Verification items for the finished model (mm, model axes). A direction names the side the tool comes from. Coordinates: 2 decimals unless noted, no trailing zeros. Write each loop counter-clockwise with the first axis right and the second up, starting at its lowest first coordinate (ties: lowest second). Pieces come first, ordered by that corner, then holes. Notation, with made-up numbers: (-21.5, 29.5) -> (-5.5, 29.5) arc R16 ccw to (-5.5, 41.5) -> close; hole circle Ø2 at (-23.5, -5). An arc over 180 degrees is marked (long way). Answer in a Markdown table with one row per item.
```python
from build123d import *

# Parameters (mm, degrees)
F0_W     = 65
F0_H     = 61
F1_DEPTH = 17.5
F2_T     = -2
F3_R     = 1.2
F4_W     = 0.8
F4_H     = 30.2
F5_DEPTH = 5
F7_DEPTH = 2


with BuildPart() as f1:
    # F0 (on Top) → F1 (new body)
    with BuildSketch(Plane.XY):
        Rectangle(F0_W, F0_H)
    extrude(amount=F1_DEPTH)

    # F2
    f2_openings = [f1.faces().sort_by_distance(p)[0] for p in [
        (0, 0, 17.5),
    ]]
    offset(amount=F2_T, openings=f2_openings)

    # F3
    f3_edges = [f1.edges().sort_by_distance(p)[0] for p in [
        (32.5, -30.5, 8.75),
        (32.5, 30.5, 8.75),
        (-32.5, 30.5, 8.75),
        (-32.5, -30.5, 8.75),
        (0, -30.5, 0),
        (-32.5, 0, 0),
        (32.5, 0, 0),
        (0, 30.5, 0),
    ]]
    fillet(f3_edges, radius=F3_R)

    # F4 (on face) → F5 (join)
    with BuildSketch(Plane.XY.offset(2)):
        Polygon((30.5, 2.5), (-30.5, 2.5), (-30.5, 1.7), (-1.3, 1.7), (-0.5, 1.7), (30.5, 1.7), align=None)
        with Locations((-0.9, -13.4)):
            Rectangle(F4_W, F4_H)
    extrude(amount=F5_DEPTH)

    # F6 (on face) → F7 (cut, through all)
    with BuildSketch(Plane(origin=(-32.5, 0, 0), x_dir=(0, -1, 0), z_dir=(-1, 0, 0))):
        Polygon((-20.3, 4.2), (-28.3, 4.2), (-27.3, 2.2), (-21.3, 2.2), align=None)
    extrude(amount=-F7_DEPTH, mode=Mode.SUBTRACT)


solid = f1.part
```
1. Depth check by flat-ended pin: P1, Ø1, axis at x = -22.5, y = 20, coming from the +Z side; P2, Ø3, axis at x = 2, y = 2.5, coming from the +Z side. Enter the tip coordinate at first touch or a pass-through.
Geometry says:
| item | result |
|---|---|
| P1 | z = 2 |
| P2 | z = 7 |
2. Mould release check, pull along Y, two halves, no side actions. Record for faces 4 (the flat face through (0, 30.5, 9)), 5 (the flat face through (0, 0, 0)), 6 (the flat face through (-31.5, 20.8, 3.2)): released by +Y, released by -Y, zero draft, split by the parting line, or undercut.
Geometry says:
| item | result |
|---|---|
| face 4 | released by +Y |
| face 5 | zero draft |
| face 6 | undercut |
3. Tool access check on faces 1 (the flat face through (0, -28.5, 10)), 2 (the flat face through (-32, 24, 4.2)), 3 (the flat face through (-32.5, 0, 9)). Record the directions out of +Z, -Z, +X, -X, +Y, -Y that give a thin tool (end or side, any length) a straight path to the whole face; none if there is none.
Geometry says:
| item | result |
|---|---|
| face 1 | +Z |
| face 2 | -X |
| face 3 | +Z, -Z, -X, +Y, -Y |
4. Section check D-D, the plane z = 11.5. Record the boundary of the cut face in (x, y).
Geometry says:
| item | result |
|---|---|
| outline | (-32.5, -29.3) arc R1.2 ccw to (-31.3, -30.5) -> (31.3, -30.5) arc R1.2 ccw to (32.5, -29.3) -> (32.5, 29.3) arc R1.2 ccw to (31.3, 30.5) -> (-31.3, 30.5) arc R1.2 ccw to (-32.5, 29.3) -> close; hole (-30.5, -28.5) -> (30.5, -28.5) -> (30.5, 28.5) -> (-30.5, 28.5) -> close |
5. Section check C-C, the plane x = -11.5. Record the boundary of the cut face in (y, z).
Geometry says:
| item | result |
|---|---|
| outline | (-30.5, 1.2) arc R1.2 ccw to (-29.3, 0) -> (29.3, 0) arc R1.2 ccw to (30.5, 1.2) -> (30.5, 17.5) -> (28.5, 17.5) -> (28.5, 2) -> (2.5, 2) -> (2.5, 7) -> (1.7, 7) -> (1.7, 2) -> (-28.5, 2) -> (-28.5, 17.5) -> (-30.5, 17.5) -> close |
6. Section check A-A, the plane z = 3. Record the boundary of the cut face in (x, y), plus the area to 3 significant figures.
Geometry says:
| item | result |
|---|---|
| outline | (-32.5, -29.3) arc R1.2 ccw to (-31.3, -30.5) -> (31.3, -30.5) arc R1.2 ccw to (32.5, -29.3) -> (32.5, 29.3) arc R1.2 ccw to (31.3, 30.5) -> (-31.3, 30.5) arc R1.2 ccw to (-32.5, 29.3) -> (-32.5, 27.7) -> (-30.5, 27.7) -> (-30.5, 28.5) -> (30.5, 28.5) -> (30.5, 2.5) -> (-30.5, 2.5) -> (-30.5, 20.9) -> (-32.5, 20.9) -> close; hole (-30.5, -28.5) -> (-1.3, -28.5) -> (-1.3, 1.7) -> (-30.5, 1.7) -> close; hole (-0.5, -28.5) -> (30.5, -28.5) -> (30.5, 1.7) -> (-0.5, 1.7) -> close |
| area | 546 mm^2 |
7. Section check B-B, the plane y = 17.5. Record the boundary of the cut face in (x, z), plus the area to 3 significant figures.
Geometry says:
| item | result |
|---|---|
| outline | (-32.5, 1.2) arc R1.2 ccw to (-31.3, 0) -> (31.3, 0) arc R1.2 ccw to (32.5, 1.2) -> (32.5, 17.5) -> (30.5, 17.5) -> (30.5, 2) -> (-30.5, 2) -> (-30.5, 17.5) -> (-32.5, 17.5) -> close |
| area | 191 mm^2 |
8. Thickness scan on line 1 (Y direction, x = -19.5, z = 4.5); line 2 (Y direction, x = -6, z = 9.5); line 3 (X direction, y = -4, z = 12.25). Record the ranges inside material, lowest first. Write a range as from..to.
Geometry says:
| item | result |
|---|---|
| line 1 | -30.5..-28.5, 1.7..2.5, 28.5..30.5 |
| line 2 | -30.5..-28.5, 28.5..30.5 |
| line 3 | -32.5..-30.5, 30.5..32.5 |
